Could you check a few things on this model? Use its own coordinates, in mm. A direction names the side the tool comes from. Round coordinates to 2 decimals unless told otherwise and drop trailing zeros. Loops run counter-clockwise (first coordinate to the right, second up) from the corner with the lowest first, then second, coordinate; pieces in that order, holes last. Notation, with made-up numbers: (-4.5, 47.25) -> (31.5, 47.25) arc R27 cw to (31.5, 75.25) -> close; hole circle Ø11 at (47, -9.5). An arc over 180 degrees is marked (long way). One line per item, written item: value.
from build123d import *

# Parameters (mm, degrees)
ESTRUSIONE_ESTRUSIONE1_DEPTH  = 12.5
TAGLIO_ESTRUSIONE1_DEPTH      = 45.229515032
TAGLIO_ESTRUSIONE1_DEPTH_BACK = 45.229515032
SCHIZZO2_W                    = 15
SCHIZZO2_H                    = 5
FORO_10_0_10_1_D              = 10
RACCORDO1_R                   = 5


with BuildPart() as part:
    # Schizzo1 → Estrusione-Estrusione1 (new, symmetric)
    with BuildSketch(Plane(origin=(0, 0, 0), x_dir=(0, 0, -1), z_dir=(1, 0, 0))):
        Polygon((0, 0), (0, 40), (10, 40), (10, 10), (30, 10), (30, 0), align=None)
    extrude(amount=ESTRUSIONE_ESTRUSIONE1_DEPTH, both=True)

    # Schizzo2 → Taglio-Estrusione1 (cut, two sides: drawn at the far end of the back side and taken through both)
    with BuildSketch(Plane(origin=(0, 10, 0), x_dir=(1, 0, 0), z_dir=(0, 1, 0)).offset(-TAGLIO_ESTRUSIONE1_DEPTH_BACK)):
        with Locations((0, 27.5)):
            Rectangle(SCHIZZO2_W, SCHIZZO2_H)
    extrude(amount=TAGLIO_ESTRUSIONE1_DEPTH + TAGLIO_ESTRUSIONE1_DEPTH_BACK, mode=Mode.SUBTRACT)

    # Foro Ø10.0 (10)-1 (through all)
    with Locations(Plane(origin=(0, 0, -10), x_dir=(-1, 0, 0), z_dir=(0, 0, -1))):
        with Locations((0, 30)):
            Hole(FORO_10_0_10_1_D / 2)

    # Raccordo1
    raccordo1_edges = [part.edges().sort_by_distance(p)[0] for p in [
        (12.5, 40, -5),
        (-12.5, 40, -5),
    ]]
    fillet(raccordo1_edges, radius=RACCORDO1_R)


solid = part.part
(1) If I drill on L1, parallel to Y at x = 0, z = -7.5; L2, parallel to Z at x = 11, y = 12; L3, parallel to Y at x = 1.25, z = -16.75, over which ranges is the centre line in solid material (lowest first)?
Recorded:
L1: 0 to 25, 35 to 40
L2: -10 to 0
L3: 0 to 10
(2) If we section it at D-D, the plane y = 4: Please give me the cut outline in (x, z), then the cut area to 3 significant figures.
Recorded:
outline: (-12.5, -30) -> (-7.5, -30) -> (-7.5, -25) -> (7.5, -25) -> (7.5, -30) -> (12.5, -30) -> (12.5, 0) -> (-12.5, 0) -> close
area: 675 mm²
(3) If we section it at A-A, the plane y = 30: Please give me the cut outline in (x, z), then the cut area to 3 significant figures.
Recorded:
outline: (-12.5, -10) -> (-5, -10) -> (-5, 0) -> (-12.5, 0) -> close; (5, -10) -> (12.5, -10) -> (12.5, 0) -> (5, 0) -> close
area: 150 mm²
(4) If we section it at C-C, the plane y = 26: Please give me the cut outline in (x, z), then the cut area to 3 significant figures.
Recorded:
outline: (-12.5, -10) -> (-3, -10) -> (-3, 0) -> (-12.5, 0) -> close; (3, -10) -> (12.5, -10) -> (12.5, 0) -> (3, 0) -> close
area: 190 mm²
(5) I'm going to push flat-ended pins straight in: pin 1 Ø10 at (x, z) = (-3.5, -19) entering from +Y; pin 2 Ø1 at (x, y) = (-1, 16.5) entering from -Z; pin 3 Ø5 at (x, y) = (-3.5, 3) entering from -Z. Where does each tip first touch, or does it pass through?
Recorded:
pin 1: y = 10
pin 2: z = -10
pin 3: z = -25
(6) If we section it at B-B, the plane x = 0: Please give me the cut outline in (y, z).
Recorded:
outline: (0, -25) -> (10, -25) -> (10, -10) -> (25, -10) -> (25, 0) -> (0, 0) -> close; (35, -10) -> (40, -10) -> (40, 0) -> (35, 0) -> close
(7) For faces 4 (the face through (12.5, 14, -9)), 5 (the face through (0, 5, -25)), 6 (the face through (0, 10, -20)), which set-ups out of +Z, -Z, +X, -X, +Y, -Y let a thin tool reach every point of the face, with its end or its side?
Recorded:
face 4: +Z, -Z, +X, +Y, -Y
face 5: -Z, +Y, -Y
face 6: -Z, +X, -X, +Y
(8) Thinking about a two-plate mould opening in X: for faces 1 (the face through (-7.5, 5, -27)), 2 (the face through (-3, 25, -10)), 3 (the face through (-11.07, 38.5, -5.07)), which applies, released by +X, released by -X, zero draft, split by the parting line, or undercut?
Recorded:
face 1: undercut
face 2: zero draft
face 3: released by -X
